Source: CAD feature listing. Evaluate the final solid. Frame: model axes, mm. A direction names the side the tool comes from. Coordinates: 2 decimals unless noted, no trailing zeros. Order: outer loops, then holes, each group sorted by start corner. A loop starts at its lowest first (then second) coordinate and runs counter-clockwise, first axis right, second up.
```python
from build123d import *

# Parameters (mm, degrees)
BOSS_EXTRUDE1_DEPTH = 2.1
SKETCH2_W           = 64.966291501
SKETCH2_H           = 1.5
BOSS_EXTRUDE2_DEPTH = 1.5


with BuildPart() as part:
    # Sketch1 → Boss-Extrude1 (new body)
    with BuildSketch(Plane(origin=(0, 0, 0), x_dir=(1, 0, 0), z_dir=(0, 1, 0))):
        with BuildLine():
            Line((4.828427125, 0), (15, 0))
            Line((15, 0), (15, 2))
            Line((15, 2), (25, 2))
            Line((25, 2), (25, 0))
            Line((25, 0), (55.78, 0))
            Line((55.78, 0), (55.78, 2))
            Line((55.78, 2), (65.78, 2))
            Line((65.78, 2), (65.78, 0))
            Line((65.78, 0), (69.794718626, 0))
            ThreePointArc((69.794718626, 0), (72.09081922, -0.456722805), (74.037359313, -1.757359313))
            Line((74.037359313, -1.757359313), (102.886601718, -30.606601718))
            ThreePointArc((102.886601718, -30.606601718), (107.75295195, -33.858192988), (113.493203436, -35))
            Line((113.493203436, -35), (162.514718626, -35))
            ThreePointArc((162.514718626, -35), (164.81081922, -35.456722805), (166.757359313, -36.757359313))
            Line((166.757359313, -36.757359313), (171.585786438, -41.585786438))
            ThreePointArc((171.585786438, -41.585786438), (172.01933194, -43.765366865), (170.171572875, -45))
            Line((170.171572875, -45), (160, -45))
            Line((160, -45), (160, -43))
            Line((160, -43), (150, -43))
            Line((150, -43), (150, -45))
            Line((150, -45), (115, -45))
            Line((115, -45), (115, -43))
            Line((115, -43), (105, -43))
            Line((105, -43), (105, -45))
            Line((105, -45), (70, -45))
            Line((70, -45), (70, -43))
            Line((70, -43), (60, -43))
            Line((60, -43), (60, -45))
            Line((60, -45), (47.485281374, -45))
            ThreePointArc((47.485281374, -45), (45.18918078, -44.543277195), (43.242640687, -43.242640687))
            Line((43.242640687, -43.242640687), (3.414213562, -3.414213562))
            ThreePointArc((3.414213562, -3.414213562), (2.98066806, -1.234633135), (4.828427125, 0))
        make_face()
        with BuildLine():
            Line((28.970562748, -10), (65.652583002, -10))
            ThreePointArc((65.652583002, -10), (67.948683596, -10.456722805), (69.895223689, -11.757359313))
            Line((69.895223689, -11.757359313), (89.723650814, -31.585786438))
            ThreePointArc((89.723650814, -31.585786438), (90.157196317, -33.765366865), (88.309437252, -35))
            Line((88.309437252, -35), (51.627416998, -35))
            ThreePointArc((51.627416998, -35), (49.331316404, -34.543277195), (47.384776311, -33.242640687))
            Line((47.384776311, -33.242640687), (27.556349186, -13.414213562))
            ThreePointArc((27.556349186, -13.414213562), (27.122803683, -11.234633135), (28.970562748, -10))
        make_face(mode=Mode.SUBTRACT)
    extrude(amount=BOSS_EXTRUDE1_DEPTH)

    # Sketch2 → Boss-Extrude2 (add)
    with BuildSketch(Plane(origin=(0, 2.1, 0), x_dir=(1, 0, 0), z_dir=(0, 1, 0))):
        with Locations((37.311572876, -0.75)):
            Rectangle(SKETCH2_W, SKETCH2_H)
    extrude(amount=BOSS_EXTRUDE2_DEPTH)


solid = part.part
```
1. Ray query, line 1 (Y direction, x = 73, z = 37); line 2 (Z direction, x = 106.5, y = 0.5); line 3 (Z direction, x = 65, y = 1.65). Return the intervals inside material, ascending.
Findings:
line 1: y = 0 to 2.1
line 2: z = 33.27 to 43
line 3: z = -2 to 10, 35 to 43
2. Section query C-C on y = 2.85. Return loops of the section in (x, z), plus the area to 3 significant figures.
Findings:
outline: (4.83, 0) - (69.79, 0) - (69.79, 1.5) - (4.83, 1.5) - close
area: 97.4 mm2
3. Access query for faces 4 (the face through (37.61, 1.04, 23.47)), 5 (the face through (107.677, 1.035, 33.826)). Directions: +Z, -Z, +X, -X, +Y, -Y. A direction counts if a zero-diameter tool reaches every point of the face in a straight line with its end or side. Return the directions, or none.
Findings:
face 4: +Y, -Y
face 5: -Z, +X, +Y, -Y
4. Draft query along Z for faces 1 (the face through (79.67, 1.04, 21.53)), 2 (the face through (24, 1, 24)), 3 (the face through (169, 1, 39)). Return one class per face: released by +Z, released by -Z, zero draft, split by the parting line, or undercut.
Findings:
face 1: undercut
face 2: released by +Z
face 3: released by -Z
5. Section query A-A on x = 67.5. Return loops of the section in (y, z), plus the area to 3 significant figures.
Findings:
outline: (0, 0) - (3.6, 0) - (3.6, 1.5) - (2.1, 1.5) - (2.1, 10.29) - (0, 10.29) - close; (0, 35) - (2.1, 35) - (2.1, 43) - (0, 43) - close
area: 40.7 mm2
6. Pin query (flat end, axial travel): P1, Ø2, axis at y = 1, z = 23.5, coming from the +X side; P2, Ø1, axis at x = 20, y = 2.5, coming from the +Z side; P3, Ø1.6, axis at y = 0.5, z = -1, coming from the -X side. Return the tip coordinate at first contact, or that it passes through.
Findings:
P1: stops at x = 96.78
P2: stops at z = 20.3
P3: stops at x = 15
7. Section query D-D on x = 157.5. Return loops of the section in (y, z).
Findings:
outline: (0, 35) - (2.1, 35) - (2.1, 43) - (0, 43) - close
8. Section query B-B on z = 20. Return loops of the section in (x, y).
Findings:
outline: (20, 0) - (34.14, 0) - (34.14, 2.1) - (20, 2.1) - close; (78.14, 0) - (92.28, 0) - (92.28, 2.1) - (78.14, 2.1) - close
